Read the model definition and answer for the solid it produces. Units are mm, in the model's axes. A direction names the side the tool comes from. Coordinates: 2 decimals unless noted, no trailing zeros. Write each loop counter-clockwise with the first axis right and the second up, starting at its lowest first coordinate (ties: lowest second). Pieces come first, ordered by that corner, then holes. Notation, with made-up numbers: (-9.75, -24) - (19.25, -24) arc R31 ccw to (19.25, 8) - close; hole circle Ø8 at (-8, 81). An arc over 180 degrees is marked (long way). Return JSON: item names as keys, results as strings.
```python
from build123d import *

# Parameters (mm, degrees)
BOSS_EXTRUDE1_DEPTH              = 6.35
SKETCH2_W                        = 203.2
SKETCH2_H                        = 6.35
BOSS_EXTRUDE2_DEPTH              = 419.1
BOSS_EXTRUDE3_DEPTH              = 6.35
F_17_64_0_26563_DIAMETER_HOLE1_D = 6.747002
F_5_32_0_15625_DIAMETER_HOLE1_D  = 3.96875
FILLET1_R                        = 6.35
CONVERT_SOLID1_START             = -101.6
CONVERT_SOLID1_DEPTH             = 203.2
CONVERT_SOLID1_2_DEPTH           = 203.2
FILLET2_R                        = 6.35


# Read off the part's stored shape, not the designer's step: Convert-Solid1
with BuildPart() as part:
    # Sketch1 → Boss-Extrude1 (new body)
    with BuildSketch(Plane(origin=(0, 0, 0), x_dir=(1, 0, 0), z_dir=(0, 1, 0))):
        Polygon((-215.9, 107.95), (-215.9, 63.5), (-101.6, 63.5), (-101.6, 50.8), (-57.15, 50.8), (-57.15, 38.1), (-101.6, 38.1), (-101.6, 0), (101.6, 0), (101.6, 38.1), (57.15, 38.1), (57.15, 50.8), (101.6, 50.8), (101.6, 63.5), (215.9, 63.5), (215.9, 107.95), align=None)
    extrude(amount=BOSS_EXTRUDE1_DEPTH)

    # Sketch2 → Boss-Extrude2 (add)
    with BuildSketch(Plane.XZ):
        with Locations((0, -3.175)):
            Rectangle(SKETCH2_W, SKETCH2_H)
    extrude(amount=BOSS_EXTRUDE2_DEPTH)

    # Sketch3 → Boss-Extrude3 (add)
    with BuildSketch(Plane.XZ.offset(419.1)):
        Polygon((-101.6, -50.8), (-101.6, -63.5), (-215.9, -63.5), (-215.9, -107.95), (215.9, -107.95), (215.9, -63.5), (101.6, -63.5), (101.6, -50.8), (57.15, -50.8), (57.15, -38.1), (101.6, -38.1), (101.6, 0), (-101.6, 0), (-101.6, -38.1), (-57.15, -38.1), (-57.15, -50.8), align=None)
    extrude(amount=BOSS_EXTRUDE3_DEPTH)

    # 17/64 (0.26563) Diameter Hole1 (through all)
    with Locations(Plane(origin=(0, 6.35, 0), x_dir=(1, 0, 0), z_dir=(0, 1, 0))):
        with Locations((-193.675, 82.55), (193.675, 82.55)):
            Hole(F_17_64_0_26563_DIAMETER_HOLE1_D / 2)

    # 5/32 (0.15625) Diameter Hole1 (through all)
    with Locations(Plane(origin=(0, 6.35, 0), x_dir=(1, 0, 0), z_dir=(0, 1, 0))):
        with Locations((-44.7675, 80.01), (-26.9875, 80.01), (26.9875, 80.01), (44.7675, 80.01)):
            Hole(F_5_32_0_15625_DIAMETER_HOLE1_D / 2)

    # Fillet1
    fillet1_edges = [part.edges().sort_by_distance(p)[0] for p in [
        (57.15, -422.275, -38.1),
        (57.15, -422.275, -50.8),
        (-57.15, -422.275, -38.1),
        (-57.15, -422.275, -50.8),
        (57.15, 3.175, -38.1),
        (57.15, 3.175, -50.8),
        (-57.15, 3.175, -38.1),
        (-57.15, 3.175, -50.8),
    ]]
    fillet(fillet1_edges, radius=FILLET1_R - 0.0001)  # a hair under: the kernel refuses the full size

    # Convert-Solid1 outline → Convert-Solid1 (cut)
    with BuildSketch(Plane.YZ.offset(CONVERT_SOLID1_START)):
        with BuildLine():
            Line((6.35, 0), (-6.35, 0))
            ThreePointArc((-6.35, 0), (2.630256121, -3.719743879), (6.35, -12.7))
            Line((6.35, -12.7), (6.35, 0))
        make_face()
        with BuildLine():
            ThreePointArc((-425.45, -12.7), (-421.730256121, -3.719743879), (-412.75, 0))
            Line((-412.75, 0), (-425.45, 0))
            Line((-425.45, 0), (-425.45, -12.7))
        make_face()
    extrude(amount=CONVERT_SOLID1_DEPTH, mode=Mode.SUBTRACT)

    # Convert-Solid1 2 outline → Convert-Solid1 2 (add)
    with BuildSketch(Plane.YZ.offset(CONVERT_SOLID1_START)):
        with BuildLine():
            Line((0, -6.35), (-6.35, -6.35))
            ThreePointArc((-6.35, -6.35), (-1.859871939, -8.209871939), (0, -12.7))
            Line((0, -12.7), (0, -6.35))
        make_face()
        with BuildLine():
            ThreePointArc((-419.1, -12.7), (-417.240128061, -8.209871939), (-412.75, -6.35))
            Line((-412.75, -6.35), (-419.1, -6.35))
            Line((-419.1, -6.35), (-419.1, -12.7))
        make_face()
    extrude(amount=CONVERT_SOLID1_2_DEPTH)

    # Fillet2
    fillet2_edges = [part.edges().sort_by_distance(p)[0] for p in [
        (101.6, 3.175, -63.5),
        (-101.6, 3.175, -63.5),
        (-101.6, -422.275, -63.5),
        (101.6, -422.275, -63.5),
    ]]
    fillet(fillet2_edges, radius=FILLET2_R)


solid = part.part
```
(1) A cutting plane is placed at A-A (x = -124). Determine the outline of the cut face in (y, z), and give its area (3 significant figures).
Answer:
{"outline": "(-425.45, -107.95) - (-419.1, -107.95) - (-419.1, -63.5) - (-425.45, -63.5) - close; (0, -107.95) - (6.35, -107.95) - (6.35, -63.5) - (0, -63.5) - close", "area": "565 mm²"}
(2) Which of the six approach directions +Z, -Z, +X, -X, +Y, -Y give full straight-line access (tool end or side, diameter ignored) to faces 4 (the face through (-1, -422, -4)), 5 (the face through (-3, 0, -72))?
Answer:
{"face 4": "+Z, +X, -X, -Y", "face 5": "-Z, +X, -X"}
(3) A cutting plane is placed at C-C (y = -317.5). Determine the outline of the cut face in (x, z), and give its area (3 significant figures).
Answer:
{"outline": "(-101.6, -6.35) - (101.6, -6.35) - (101.6, 0) - (-101.6, 0) - close", "area": "1,290 mm²"}
(4) Flat-ended cylindrical pins translate along their axes: P1, Ø5, axis at x = -139.5, y = 4.5, coming from the +Z side; P2, Ø6.5, axis at x = 44.77, z = -80.01, coming from the -Y side; P3, Ø5, axis at x = 82, y = -420.5, coming from the +Z side; P4, Ø6, axis at x = -193.675, z = -82.55, coming from the -Y side. Find the tip coordinate at first contact, or state that the pin passes through.
Answer:
{"P1": "z = -63.5", "P2": "y = -425.45", "P3": "z = -1.14", "P4": "through"}
(5) A cutting plane is placed at B-B (z = -23.5). Determine the outline of the cut face in (x, y).
Answer:
{"outline": "(-101.6, -425.45) - (101.6, -425.45) - (101.6, -419.1) - (-101.6, -419.1) - close; (-101.6, 0) - (101.6, 0) - (101.6, 6.35) - (-101.6, 6.35) - close"}
(6) Determine the mould class of faces 1 (the face through (-101.6, -211, -3)), 2 (the face through (-3, -419.1, -70)), 3 (the face through (-3, 6.35, -72)) for opening direction Y: +Y half, -Y half, draft (parallel to the pull), parting line (faces both ways), or undercut.
Answer:
{"face 1": "draft", "face 2": "undercut", "face 3": "+Y half"}
(7) Straight lines are drawn through the part: line 1 (Y direction, x = -75, z = -20); line 2 (Z direction, x = 91.5, y = -15.5); line 3 (X direction, y = -183, z = -4.5). For each, find the intervals that lie inside material, in ascending order. Write a range as from..to.
Answer:
{"line 1": "-425.45..-419.1, 0..6.35", "line 2": "-6.35..0", "line 3": "-101.6..101.6"}
